Model file for the job. Use its own axes, mm. Round coordinates to 2 decimals unless told otherwise and drop trailing zeros. Loops run counter-clockwise (first coordinate to the right, second up) from the corner with the lowest first, then second, coordinate; pieces in that order, holes last. Notation, with made-up numbers: M -26.5,67.5 L 7.5,67.5 A23 ccw 7.5,104.5 Z; hole C -16,1 d7. An arc over 180 degrees is marked long. Use a Markdown table: item, result. Add a question column.
Item 1: Saw through at D-D on x = -37.5. Give the number of separate pieces and of enclosed holes in the cut face, then the cut area to 3 significant figures.
Item 2: Saw through at B-B on x = 41. Write the cut outline in (y, z) (3 decimals), then the cut area to 4 significant figures.
Item 3: Saw through at A-A on z = 16. Write the cut outline in (x, y) (3 decimals).
Item 4: Wall check: L1, parallel to Z at x = -37.5, y = 1.2 (3 decimals); L2, parallel to Z at x = 41, y = 1 (3 decimals); L3, parallel to Y at x = 22, z = -1.5. Give the ranges that are in metal, low to high. Write a range as from..to.
Item 5: Saw through at C-C on y = 1.05. Write the cut outline in (x, z) (3 decimals).
Item 6: Pin check, flat tips, straight feed: P1, Ø3.5, axis at x = 41, z = 16, coming from the -Y side; P2, Ø5, axis at x = -0.5, z = -12, coming from the +Y side. Stop position of each tip, or through.
```python
from build123d import *

# Parameters (mm, degrees)
SKETCH1_W                = 86.5
SKETCH1_H                = 40
BOSS_EXTRUDE1_DEPTH      = 1.5
SKETCH2_W                = 7.62
SKETCH2_H                = 5.0978
CUT_EXTRUDE1_DEPTH       = 2.5
CHAMFER2_SIZE            = 1.5
SKETCH4_R                = 1.625
CUT_EXTRUDE2_DEPTH       = 2.5
SKETCH3_W                = 7
SKETCH3_H                = 1.651
BOSS_EXTRUDE2_DEPTH      = 0.05
BOSS_EXTRUDE2_DEPTH_BACK = 1.55


with BuildPart() as part:
    # Sketch1 → Boss-Extrude1 (new body)
    with BuildSketch(Plane(origin=(0, 0, 0), x_dir=(1, 0, 0), z_dir=(0, 1, 0))):
        with Locations((1.75, 0)):
            Rectangle(SKETCH1_W, SKETCH1_H)
    extrude(amount=BOSS_EXTRUDE1_DEPTH)

    # Sketch2 → Cut-Extrude1 (cut, through all)
    with BuildSketch(Plane(origin=(0, 1.5, 0), x_dir=(1, 0, 0), z_dir=(0, 1, 0))):
        with Locations((-37.69, 5.4511)):
            Rectangle(SKETCH2_W, SKETCH2_H)
        with Locations((-37.69, -9.4511)):
            Rectangle(SKETCH2_W, SKETCH2_H)
    extrude(amount=-CUT_EXTRUDE1_DEPTH, mode=Mode.SUBTRACT)

    # Chamfer2
    chamfer2_edges = [part.edges().sort_by_distance(p)[0] for p in [
        (-41.5, 0.75, -2.9022),
        (-41.5, 0.75, -8),
        (-33.88, 0.75, -8),
        (-41.5, 0.75, 12),
        (-41.5, 0.75, 6.9022),
        (-33.88, 0.75, 12),
        (-41.5, 0.75, -20),
        (-41.5, 0.75, 20),
    ]]
    chamfer(chamfer2_edges, length=CHAMFER2_SIZE)

    # Sketch4 → Cut-Extrude2 (cut, through all)
    with BuildSketch(Plane.XZ):
        with Locations((-37.5, 16)):
            Circle(SKETCH4_R)
        with Locations((41, 16)):
            Circle(SKETCH4_R)
        with Locations((41, -16)):
            Circle(SKETCH4_R)
        with Locations((-37.5, -16)):
            Circle(SKETCH4_R)
    extrude(amount=-CUT_EXTRUDE2_DEPTH, mode=Mode.SUBTRACT)

    # Sketch3 → Boss-Extrude2 (add, two sides)
    with BuildSketch(Plane(origin=(0, 1.5, 0), x_dir=(1, 0, 0), z_dir=(0, 1, 0))) as boss_extrude2_sk:
        with Locations((-38, 0.54)):
            Rectangle(SKETCH3_W, SKETCH3_H)
        with Locations((-38, -2)):
            Rectangle(SKETCH3_W, SKETCH3_H)
        with Locations((-38, -4.54)):
            Rectangle(SKETCH3_W, SKETCH3_H)
    extrude(amount=BOSS_EXTRUDE2_DEPTH)
    extrude(boss_extrude2_sk.sketch, amount=-BOSS_EXTRUDE2_DEPTH_BACK)


solid = part.part
```
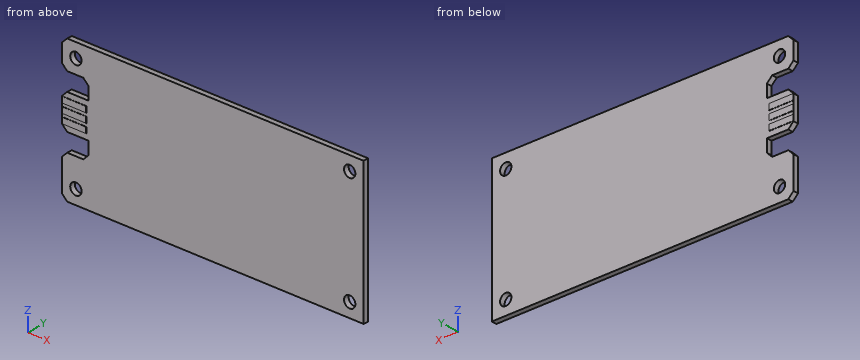
Entries:
| question | item | result |
|---|---|---|
| 1 | separate pieces | 5 |
| 1 | enclosed holes | 0 |
| 1 | area | 35.5 mm2 |
| 2 | outline | M 0,-20 L 1.5,-20 L 1.5,-17.625 L 0,-17.625 Z; M 0,-14.375 L 1.5,-14.375 L 1.5,14.375 L 0,14.375 Z; M 0,17.625 L 1.5,17.625 L 1.5,20 L 0,20 Z |
| 2 | area | 50.25 mm2 |
| 3 | outline | M -41.5,0 L -39.125,0 L -39.125,1.5 L -41.5,1.5 Z; M -35.875,0 L 39.375,0 L 39.375,1.5 L -35.875,1.5 Z; M 42.625,0 L 45,0 L 45,1.5 L 42.625,1.5 Z |
| 4 | L1 | -20..-17.625, -14.375..-8, -2.902..6.902, 12..14.375, 17.625..20 |
| 4 | L2 | -20..-17.625, -14.375..14.375, 17.625..20 |
| 4 | L3 | 0..1.5 |
| 5 | outline | M -41.5,-18.5 L -40,-20 L 45,-20 L 45,20 L -40,20 L -41.5,18.5 L -41.5,13.5 L -40,12 L -35.38,12 L -33.88,10.5 L -33.88,6.902 L -40,6.902 L -41.5,5.402 L -41.5,-1.402 L -40,-2.902 L -33.88,-2.902 L -33.88,-6.5 L -35.38,-8 L -40,-8 L -41.5,-9.5 Z; hole C -37.5,-16 d3.25; hole C -37.5,16 d3.25; hole C 41,-16 d3.25; hole C 41,16 d3.25 |
| 6 | P1 | y = 0 |
| 6 | P2 | y = 1.5 |
